Geometry check sheet. Reference: the model listing, model coordinates, mm. Face numbers are marked on the shaded views. A direction names the side the tool comes from. Round coordinates to 2 decimals unless told otherwise and drop trailing zeros. Write each loop counter-clockwise with the first axis right and the second up, starting at its lowest first coordinate (ties: lowest second). Pieces come first, ordered by that corner, then holes.
Item 1: Draft check along Z on the marked faces 1, 2 and 3. Enter one of: pulls with the +Z half, pulls with the -Z half, needs draft (parallel to the pull), parting line crosses it, or undercut.
Item 2: Cross-section at A-A (x = 69). Enter the section's corners in (y, z).
Item 3: Scan lines: probe 1 along Z at (x, y) = (173, -2); probe 2 along X at (y, z) = (-1.25, -168); probe 3 along X at (y, z) = (16, -156.5). Record each from-to range of solid material in increasing order.
Item 4: Depth check by flat-ended pin: P1, Ø5, axis at x = 173, z = -168, coming from the +Y side; P2, Ø3.5, axis at x = 110, z = -217, coming from the +Y side. Enter the tip coordinate at first touch or a pass-through.
Item 5: Access from +Z, -Z, +X, -X, +Y, -Y to the whole of each face (thin tool, end or side, straight path). Record for the marked faces 4 and 5.
Item 6: Cross-section at B-B (z = -150.5). Enter the section's corners in (x, y).
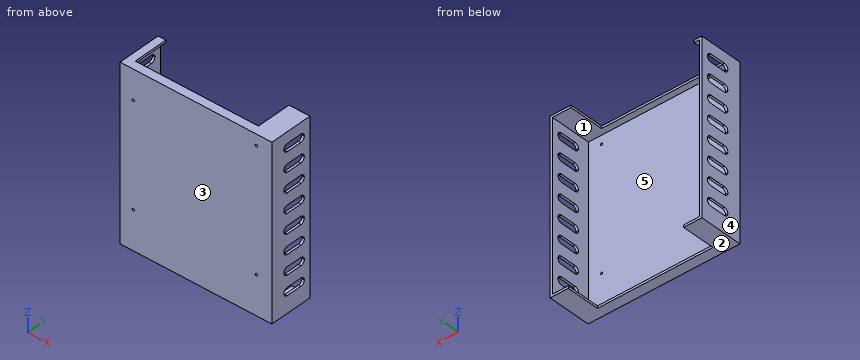
from build123d import *

# Parameters (mm, degrees)
SKETCH_2_W          = 196
SKETCH_2_H          = 221
SKETCH_2_R          = 1.5
EXTRUDE_8_DEPTH     = 3
SKETCH_1_W          = 196
SKETCH_1_H          = 221
SKETCH_1_W_2        = 190
SKETCH_1_H_2        = 215
EXTRUDE_9_DEPTH     = 8
EXTRUDE_10_DEPTH    = 45
CUT_EXTRUDE_1_DEPTH = 5
CUT_EXTRUDE_2_DEPTH = 209


with BuildPart() as part:
    # 草图2 → 凸台-拉伸8 (new body)
    with BuildSketch(Plane(origin=(0, -3, 0), x_dir=(1, 0, 0), z_dir=(0, 1, 0))):
        with Locations((95, 107.5)):
            Rectangle(SKETCH_2_W, SKETCH_2_H)
        with Locations((14, 168)):
            Circle(SKETCH_2_R, mode=Mode.SUBTRACT)
        with Locations((173, 168)):
            Circle(SKETCH_2_R, mode=Mode.SUBTRACT)
        with Locations((173, 11)):
            Circle(SKETCH_2_R, mode=Mode.SUBTRACT)
        with Locations((14, 35)):
            Circle(SKETCH_2_R, mode=Mode.SUBTRACT)
    extrude(amount=EXTRUDE_8_DEPTH)

    # 草图1 → 凸台-拉伸9 (add)
    with BuildSketch(Plane(origin=(0, 0, 0), x_dir=(1, 0, 0), z_dir=(0, 1, 0))):
        with Locations((95, 107.5)):
            Rectangle(SKETCH_1_W, SKETCH_1_H)
        with Locations((95, 107.5)):
            Rectangle(SKETCH_1_W_2, SKETCH_1_H_2, mode=Mode.SUBTRACT)
    extrude(amount=EXTRUDE_9_DEPTH)

    # 草图9 → 凸台-拉伸10 (add)
    with BuildSketch(Plane(origin=(0, 8, 0), x_dir=(1, 0, 0), z_dir=(0, 1, 0))):
        Polygon((166, -3), (193, -3), (193, 218), (-3, 218), (-3, -3), (7, -3), (7, 0), (0, 0), (0, 215), (190, 215), (190, 0), (166, 0), align=None)
    extrude(amount=EXTRUDE_10_DEPTH)

    # 草图10 → 切除-拉伸1 (cut)
    with BuildSketch(Plane(origin=(0, 0, -218), x_dir=(-1, 0, 0), z_dir=(0, 0, -1))):
        Polygon((-95, 10), (-169.5, 10), (-169.5, 53), (-20.5, 53), (-20.5, 10), align=None)
    extrude(amount=-CUT_EXTRUDE_1_DEPTH, mode=Mode.SUBTRACT)

    # 草图11 → 切除-拉伸2 (cut)
    with BuildSketch(Plane(origin=(193, 0, 0), x_dir=(0, 0, -1), z_dir=(1, 0, 0))):
        with BuildLine():
            Line((196.326880945, 39.740756609), (196.326880945, 19.740756609))
            ThreePointArc((196.326880945, 19.740756609), (194.862414851, 16.205222703), (191.326880945, 14.740756609))
            ThreePointArc((191.326880945, 14.740756609), (187.791347039, 16.205222703), (186.326880945, 19.740756609))
            Line((186.326880945, 19.740756609), (186.326880945, 39.740756609))
            ThreePointArc((186.326880945, 39.740756609), (187.791347039, 43.276290515), (191.326880945, 44.740756609))
            ThreePointArc((191.326880945, 44.740756609), (194.862414851, 43.276290515), (196.326880945, 39.740756609))
        make_face()
        with BuildLine():
            Line((36.326880945, 39.740756609), (36.326880945, 19.740756609))
            ThreePointArc((36.326880945, 19.740756609), (37.791347039, 16.205222703), (41.326880945, 14.740756609))
            ThreePointArc((41.326880945, 14.740756609), (44.862414851, 16.205222703), (46.326880945, 19.740756609))
            Line((46.326880945, 19.740756609), (46.326880945, 39.740756609))
            ThreePointArc((46.326880945, 39.740756609), (44.862414851, 43.276290515), (41.326880945, 44.740756609))
            ThreePointArc((41.326880945, 44.740756609), (37.791347039, 43.276290515), (36.326880945, 39.740756609))
        make_face()
        with BuildLine():
            Line((11.326880945, 39.740756609), (11.326880945, 19.740756609))
            ThreePointArc((11.326880945, 19.740756609), (12.791347039, 16.205222703), (16.326880945, 14.740756609))
            ThreePointArc((16.326880945, 14.740756609), (19.862414851, 16.205222703), (21.326880945, 19.740756609))
            Line((21.326880945, 19.740756609), (21.326880945, 39.740756609))
            ThreePointArc((21.326880945, 39.740756609), (19.862414851, 43.276290515), (16.326880945, 44.740756609))
            ThreePointArc((16.326880945, 44.740756609), (12.791347039, 43.276290515), (11.326880945, 39.740756609))
        make_face()
        with BuildLine():
            Line((61.326880945, 39.740756609), (61.326880945, 19.740756609))
            ThreePointArc((61.326880945, 19.740756609), (62.791347039, 16.205222703), (66.326880945, 14.740756609))
            ThreePointArc((66.326880945, 14.740756609), (69.862414851, 16.205222703), (71.326880945, 19.740756609))
            Line((71.326880945, 19.740756609), (71.326880945, 39.740756609))
            ThreePointArc((71.326880945, 39.740756609), (69.862414851, 43.276290515), (66.326880945, 44.740756609))
            ThreePointArc((66.326880945, 44.740756609), (62.791347039, 43.276290515), (61.326880945, 39.740756609))
        make_face()
        with BuildLine():
            Line((86.326880945, 39.740756609), (86.326880945, 19.740756609))
            ThreePointArc((86.326880945, 19.740756609), (87.791347039, 16.205222703), (91.326880945, 14.740756609))
            ThreePointArc((91.326880945, 14.740756609), (94.862414851, 16.205222703), (96.326880945, 19.740756609))
            Line((96.326880945, 19.740756609), (96.326880945, 39.740756609))
            ThreePointArc((96.326880945, 39.740756609), (94.862414851, 43.276290515), (91.326880945, 44.740756609))
            ThreePointArc((91.326880945, 44.740756609), (87.791347039, 43.276290515), (86.326880945, 39.740756609))
        make_face()
        with BuildLine():
            Line((111.326880945, 39.740756609), (111.326880945, 19.740756609))
            ThreePointArc((111.326880945, 19.740756609), (112.791347039, 16.205222703), (116.326880945, 14.740756609))
            ThreePointArc((116.326880945, 14.740756609), (119.862414851, 16.205222703), (121.326880945, 19.740756609))
            Line((121.326880945, 19.740756609), (121.326880945, 39.740756609))
            ThreePointArc((121.326880945, 39.740756609), (119.862414851, 43.276290515), (116.326880945, 44.740756609))
            ThreePointArc((116.326880945, 44.740756609), (112.791347039, 43.276290515), (111.326880945, 39.740756609))
        make_face()
        with BuildLine():
            Line((136.326880945, 39.740756609), (136.326880945, 19.740756609))
            ThreePointArc((136.326880945, 19.740756609), (137.791347039, 16.205222703), (141.326880945, 14.740756609))
            ThreePointArc((141.326880945, 14.740756609), (144.862414851, 16.205222703), (146.326880945, 19.740756609))
            Line((146.326880945, 19.740756609), (146.326880945, 39.740756609))
            ThreePointArc((146.326880945, 39.740756609), (144.862414851, 43.276290515), (141.326880945, 44.740756609))
            ThreePointArc((141.326880945, 44.740756609), (137.791347039, 43.276290515), (136.326880945, 39.740756609))
        make_face()
        with BuildLine():
            Line((161.326880945, 39.740756609), (161.326880945, 19.740756609))
            ThreePointArc((161.326880945, 19.740756609), (162.791347039, 16.205222703), (166.326880945, 14.740756609))
            ThreePointArc((166.326880945, 14.740756609), (169.862414851, 16.205222703), (171.326880945, 19.740756609))
            Line((171.326880945, 19.740756609), (171.326880945, 39.740756609))
            ThreePointArc((171.326880945, 39.740756609), (169.862414851, 43.276290515), (166.326880945, 44.740756609))
            ThreePointArc((166.326880945, 44.740756609), (162.791347039, 43.276290515), (161.326880945, 39.740756609))
        make_face()
    extrude(amount=-CUT_EXTRUDE_2_DEPTH, mode=Mode.SUBTRACT)


solid = part.part
Resolved:
1. face 1: undercut
1. face 2: pulls with the -Z half
1. face 3: needs draft
2. outline: (-3, -218) - (10, -218) - (10, -215) - (0, -215) - (0, 0) - (8, 0) - (8, 3) - (-3, 3) - close
3. probe 1: z = -218 to -169.5, -166.5 to -12.5, -9.5 to 3
3. probe 2: x = -3 to 12.5, 15.5 to 171.5, 174.5 to 193
3. probe 3: x = -3 to 0, 190 to 193
4. P1: stops at y = 0
4. P2: stops at y = 10
5. face 4: +Z, -Z, -X, +Y, -Y
5. face 5: +Y
6. outline: (-3, -3) - (193, -3) - (193, 53) - (190, 53) - (190, 0) - (0, 0) - (0, 53) - (-3, 53) - close
